from build123d import *

# Parameters (mm, degrees)
CUT_EXTRUDE1_DEPTH      = 20.05
CUT_EXTRUDE1_DEPTH_BACK = 20.05
CUT_EXTRUDE2_DEPTH      = 20.05
CUT_EXTRUDE2_DEPTH_BACK = 20.05
SKETCH4_R               = 0.79375


with BuildPart() as part:
    # Sketch2 → Revolve1 (revolve)
    with BuildSketch(Plane.XY, mode=Mode.PRIVATE) as revolve1_sk:
        Polygon((0, 0), (0, 12.7), (1.5875, 12.7), (3.175, 6.35), (4.7625, 12.7), (6.35, 12.7), (6.35, 0), align=None)
    revolve(revolve1_sk.sketch.rotate(Axis((0, 0, 0), (1, 0, 0)), 90), axis=Axis((0, 0, 0), (1, 0, 0)))

    # Sketch3 → Cut-Extrude1 (cut, two sides: drawn at the far end of the back side and taken through both)
    with BuildSketch(Plane(origin=(6.35, 0, 0), x_dir=(0, 0, -1), z_dir=(1, 0, 0)).offset(-CUT_EXTRUDE1_DEPTH_BACK)):
        with BuildLine():
            Line((2.392934, -1.80937306), (2.392934, 1.80937306))
            ThreePointArc((2.392934, 1.80937306), (-2.999994, 0), (2.392934, -1.80937306))
        make_face()
    extrude(amount=CUT_EXTRUDE1_DEPTH + CUT_EXTRUDE1_DEPTH_BACK, mode=Mode.SUBTRACT)

    # Sketch4 → Cut-Extrude2 (cut, two sides: drawn at the far end of the back side and taken through both)
    with BuildSketch(Plane(origin=(6.35, 0, 0), x_dir=(0, 0, -1), z_dir=(1, 0, 0)).offset(-CUT_EXTRUDE2_DEPTH_BACK)):
        with Locations((-9.525, 0)):
            Circle(SKETCH4_R)
    extrude(amount=CUT_EXTRUDE2_DEPTH + CUT_EXTRUDE2_DEPTH_BACK, mode=Mode.SUBTRACT)


solid = part.part
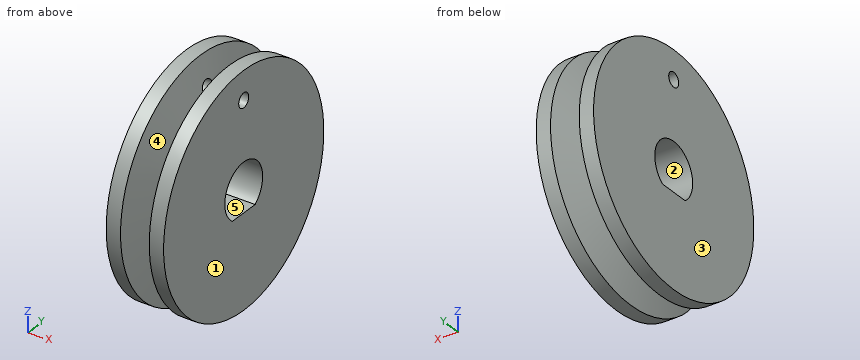
For this review, take the finished solid that the model builds, in its own axes (mm). Face numbers are marked on the shaded views. A direction names the side the tool comes from. Round coordinates to 2 decimals unless told otherwise and drop trailing zeros. Order: outer loops, then holes, each group sorted by start corner. A loop starts at its lowest first (then second) coordinate and runs counter-clockwise, first axis right, second up. Notation, with made-up numbers: (80, 45) -> (134, 45) arc R10 ccw to (134, 49) -> close; hole circle Ø7 at (56.5, -37.75). An arc over 180 degrees is marked (long way). Put each result on its own line as item: value.
Q1. Add section B-B on y = 0. State how many separate pieces and enclosed holes the cut face has, plus the area to 3 significant figures.
Check result:
separate pieces: 4
enclosed holes: 0
area: 99.3 mm2
Q2. Machinability: for the marked faces 3, 4 and 5, which of the approach directions +Z, -Z, +X, -X, +Y, -Y give a long, thin tool a straight path to every point of the face, cutting with its end or side? Answer none if there is none.
Check result:
face 3: +Z, -Z, -X, +Y, -Y
face 4: none
face 5: +X, -X
Q3. Insertion check: pin 1 Ø3 at (x, y) = (2.5, 1) entering from +Z; pin 2 Ø1 at (y, z) = (0, 9.525) entering from +X; pin 3 Ø1 at (x, y) = (5.5, 4.5) entering from -Z. Each pin has a flat end and moves straight along its axis. Give the tip position at first contact, or say it passes through.
Check result:
pin 1: z = 12.7
pin 2: through
pin 3: z = -12.05
Q4. Add section C-C on x = 6. Write out the cut boundary in (y, z) (1 decimal), plus the area to 3 significant figures.
Check result:
outline: circle Ø25.4 at (0, 0); hole (-1.8, -2.4) -> (1.8, -2.4) arc R3 ccw (long way) to start; hole circle Ø1.6 at (0, 9.5)
area: 478 mm2
Q5. Mouldability with a two-part tool opening along Z and no side actions: class the marked faces 1 and 2 as pulls with the +Z half, pulls with the -Z half, needs draft (parallel to the pull), parting line crosses it, or undercut.
Check result:
face 1: needs draft
face 2: undercut
Q6. For probe 1 along Y at (x, z) = (5.25, 0); probe 2 along X at (y, z) = (-5, 6.25); probe 3 along X at (y, z) = (-7, -7.25), list the stretches that pass through material, from the lowest coordinate up. Write a range as [from, to].
Check result:
probe 1: [-12.7, -3], [3, 12.7]
probe 2: [0, 2.76], [3.59, 6.35]
probe 3: [0, 2.24], [4.11, 6.35]
